For this review, use the dimensioned drawing (mm, ordinates from the lowest corner) and the shaded views. A direction names the side the tool comes from. Round coordinates to 2 decimals unless told otherwise and drop trailing zeros. Write each loop counter-clockwise with the first axis right and the second up, starting at its lowest first coordinate (ties: lowest second). Pieces come first, ordered by that corner, then holes. Notation, with made-up numbers: (11, 40) -> (17, 40) arc R6 cw to (17, 49) -> close; hole circle Ø9 at (-3.75, 25.25). An arc over 180 degrees is marked (long way). Write each question's results on one line, items separated by ' | '. Start each with the question number.
Item 1: Add section A-A (x = 2.2). State the section outline as (y, z) points.
Item 2: Clearance check with flat-ended pins moving along their axes: pin 1 (1 mm diameter, centred on x = 15, z = 2.5, fed in from +Y); pin 2 (1 mm diameter, centred on x = 29, z = 5.5, fed in from +Y); pin 3 (1.6 mm diameter, centred on x = 4, z = 4, fed in from -Y). State where each tip first meets the part, or that it passes through.
Item 3: Add section C-C (x = 21). State the section outline as (y, z) points, plus the area to 3 significant figures.
Item 4: Tool access review of the marked faces 1, 2 and 3: name each direction out of +Z, -Z, +X, -X, +Y, -Y from which nothing blocks a thin tool from reaching the whole face with its end or side.
Item 5: Add section D-D (y = 24.5). State the section outline as (x, z) points, plus the area to 3 significant figures.
Item 6: To check wall thickness, follow line 1 along Z through (x, y) = (21, 27.75); line 2 along X through (y, z) = (12, 2.5); line 3 along Y through (x, z) = (4, 11.25). State the ranges of each line that lie inside material, in increasing order.
Item 7: Add section B-B (z = 5.9). State the section outline as (x, y) points, plus the area to 3 significant figures.
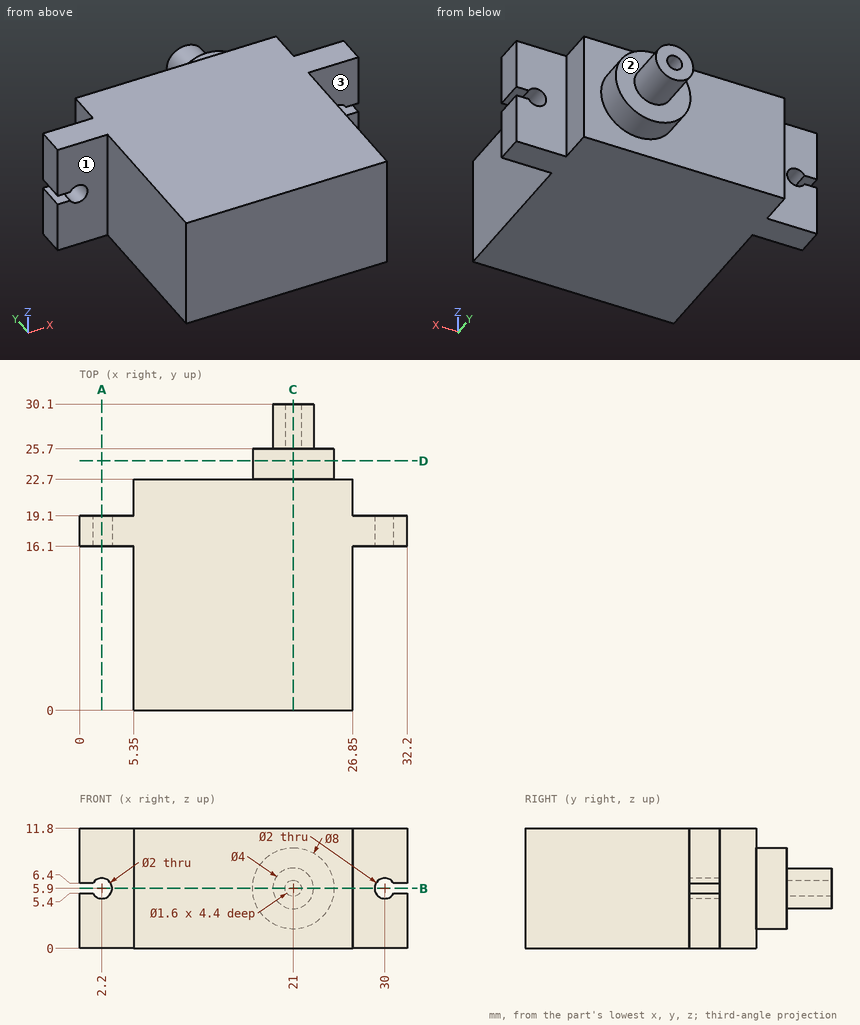
Responses:
1) outline: (16.1, 0) -> (19.1, 0) -> (19.1, 4.9) -> (16.1, 4.9) -> close; (16.1, 6.9) -> (19.1, 6.9) -> (19.1, 11.8) -> (16.1, 11.8) -> close
2) pin 1: stops at y = 22.7 | pin 2: stops at y = 19.1 | pin 3: stops at y = 16.1
3) outline: (0, 0) -> (22.7, 0) -> (22.7, 1.9) -> (25.7, 1.9) -> (25.7, 3.9) -> (30.1, 3.9) -> (30.1, 5.1) -> (25.7, 5.1) -> (25.7, 6.7) -> (30.1, 6.7) -> (30.1, 7.9) -> (25.7, 7.9) -> (25.7, 9.9) -> (22.7, 9.9) -> (22.7, 11.8) -> (0, 11.8) -> close | area: 302 mm^2
4) face 1: +Z, -Z, -X, -Y | face 2: +Y | face 3: +Z, -Z, +X, -Y
5) outline: circle Ø8 at (21, 5.9) | area: 50.3 mm^2
6) line 1: z = 3.9 to 5.1, 6.7 to 7.9 | line 2: x = 5.35 to 26.85 | line 3: y = 16.1 to 19.1
7) outline: (3.2, 16.1) -> (5.35, 16.1) -> (5.35, 0) -> (26.85, 0) -> (26.85, 16.1) -> (29, 16.1) -> (29, 19.1) -> (26.85, 19.1) -> (26.85, 22.7) -> (25, 22.7) -> (25, 25.7) -> (23, 25.7) -> (23, 30.1) -> (21.8, 30.1) -> (21.8, 25.7) -> (20.2, 25.7) -> (20.2, 30.1) -> (19, 30.1) -> (19, 25.7) -> (17, 25.7) -> (17, 22.7) -> (5.35, 22.7) -> (5.35, 19.1) -> (3.2, 19.1) -> close | area: 536 mm^2
